For this review, take the finished solid that the model builds, in its own axes (mm). Give positions to 0.01 mm unless a question says otherwise; leave off trailing zeros. Write each loop counter-clockwise with the first axis right and the second up, starting at its lowest first coordinate (ties: lowest second). Pieces come first, ordered by that corner, then holes. Notation, with made-up numbers: (-15.5, -6.75) -> (20.5, -6.75) arc R24 ccw to (20.5, 30.25) -> close; hole circle Ø1 at (29, 63.25). An arc over 180 degrees is marked (long way). Answer as CSV lines item,"result".
```python
from build123d import *

# Parameters (mm, degrees)
SKETCH1_W           = 6
SKETCH1_H           = 6
BOSS_EXTRUDE1_DEPTH = 3
CHAMFER1_SIZE       = 0.5


with BuildPart() as part:
    # Sketch1 → Boss-Extrude1 (new, symmetric)
    with BuildSketch(Plane(origin=(0, 0, 0), x_dir=(1, 0, 0), z_dir=(0, 1, 0))):
        Rectangle(SKETCH1_W, SKETCH1_H)
    extrude(amount=BOSS_EXTRUDE1_DEPTH, both=True)

    # Chamfer1
    chamfer1_edges = [part.edges().sort_by_distance(p)[0] for p in [
        (-3, 3, 0),
        (0, 3, 3),
        (3, 3, 0),
        (0, -3, 3),
        (-3, -3, 0),
        (0, -3, -3),
        (3, -3, 0),
        (3, 0, 3),
        (-3, 0, 3),
        (-3, 0, -3),
        (3, 0, -3),
        (0, 3, -3),
    ]]
    chamfer(chamfer1_edges, length=CHAMFER1_SIZE)


solid = part.part
```
Q1. Add section A-A (x = 2.6). Write out the cut boundary in (y, z).
Answer block:
outline,"(-2.9, -2.5) -> (-2.5, -2.9) -> (2.5, -2.9) -> (2.9, -2.5) -> (2.9, 2.5) -> (2.5, 2.9) -> (-2.5, 2.9) -> (-2.9, 2.5) -> close"
Q2. To check wall thickness, follow probe 1 along Z at (x, y) = (2.7, -2.45). State the ranges of the line that lie inside material, in increasing order. Write a range as [from, to].
Answer block:
probe 1,"z = [-2.8, 2.8]"
